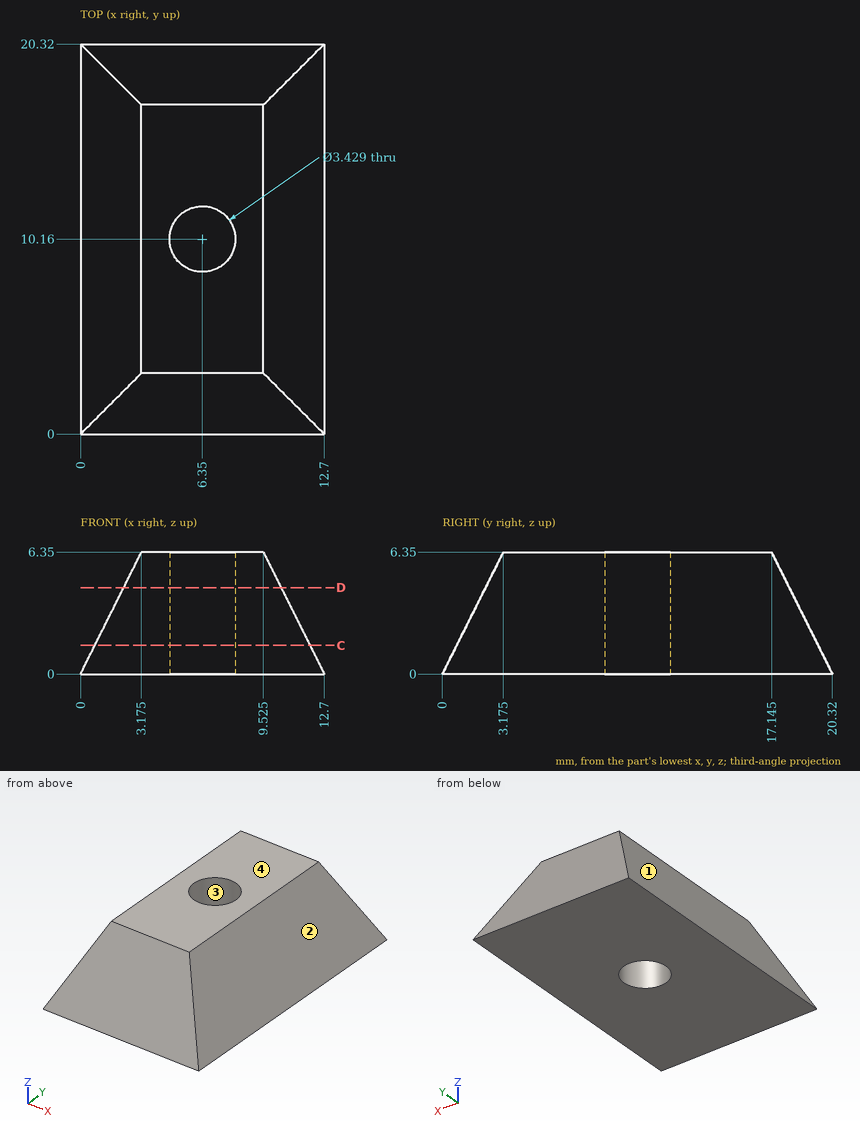
Geometry check sheet. Reference: drawing and pictorial views, mm from the part's lowest x, y, z. Coordinates: 2 decimals unless noted, no trailing zeros. Order: outer loops, then holes, each group sorted by start corner. A loop starts at its lowest first (then second) coordinate and runs counter-clockwise, first axis right, second up. Notation, with made-up numbers: (-36.75, 13.25) -> (22.25, 13.25) arc R16 cw to (22.25, 24.25) -> close; hole circle Ø4 at (81.5, -27.5). An arc over 180 degrees is marked (long way). Put each result on its own line as item: value. Start each with the question number.
1) Release check for a two-part mould opening along X. For the marked faces 1, 2, 3 and 4 record: pulls with the +X half, pulls with the -X half, needs draft (parallel to the pull), parting line crosses it, or undercut.
2) Material ranges on L1, parallel to Y at x = 6, z = 1.75 (3 decimals); L2, parallel to Y at x = 6.35, z = 3.25 (1 decimal); L3, parallel to X at y = 9.5, z = 2.25 (3 decimals), recorded low to high.
3) Go/stop test with flat-tipped pins: pin 1 (1.5 mm diameter, centred on x = 1.5, z = 1, fed in from -Y) (3 decimals); pin 2 (2 mm diameter, centred on x = 2, z = 3.5, fed in from -Y); pin 3 (2 mm diameter, centred on x = 11, y = 8.5, fed in from +Z). Record where each tip stops, or that it passes through.
4) Cross-section at D-D (z = 4.5). Enter the section's corners in (x, y).
5) Cross-section at C-C (z = 1.5). Enter the section's corners in (x, y).
Geometry check:
1. face 1: pulls with the -X half
1. face 2: pulls with the +X half
1. face 3: undercut
1. face 4: needs draft
2. L1: y = 0.875 to 8.482, 11.838 to 19.445
2. L2: y = 1.6 to 8.4, 11.9 to 18.7
2. L3: x = 1.125 to 4.768, 7.932 to 11.575
3. pin 1: stops at y = 0.125
3. pin 2: stops at y = 1.25
3. pin 3: stops at z = 5.4
4. outline: (2.25, 2.25) -> (10.45, 2.25) -> (10.45, 18.07) -> (2.25, 18.07) -> close; hole circle Ø3.43 at (6.35, 10.16)
5. outline: (0.75, 0.75) -> (11.95, 0.75) -> (11.95, 19.57) -> (0.75, 19.57) -> close; hole circle Ø3.43 at (6.35, 10.16)
